The model under review builds one solid part; all positions refer to its coordinate system, in mm. A direction names the side the tool comes from. Coordinates: 2 decimals unless noted, no trailing zeros. Loops run counter-clockwise (first coordinate to the right, second up) from the corner with the lowest first, then second, coordinate; pieces in that order, holes last. Notation, with made-up numbers: M 58.25,49.25 L 80.25,49.25 A23 ccw 80.25,57.25 Z; hole C 27.25,16.25 d7. An arc over 180 degrees is marked long. Use CSV: the item, a comma, the result in double quotes. Start each with the question number.
1. Tool access review of faces 1 (the flat face through (7, 7, 0)), 2 (the flat face through (0.125, -11, 3)): name each direction out of +Z, -Z, +X, -X, +Y, -Y from which nothing blocks a thin tool from reaching the whole face with its end or side.
2. For L1, parallel to X at y = -5.25, z = 2.6; L2, parallel to Y at x = 3.5, z = 0.6; L3, parallel to X at y = 0, z = 1 (3 decimals), list the stretches that pass through material, from the lowest coordinate up.
3. Clearance check with flat-ended pins moving along their axes: P1, Ø9.5, axis at x = 2.5, y = -2, coming from the +Z side; P2, Ø1, axis at y = -7.5, z = 2, coming from the -X side; P3, Ø2.5, axis at y = -11, z = 1.5, coming from the +X side; P4, Ø2.5, axis at y = -11, z = 3, coming from the -X side. State where each tip first meets the part, or that it passes through.
4. Add section A-A, the plane z = 1.2. Write out the cut boundary in (x, y) (3 decimals), then the cut area to 3 significant figures.
from build123d import *

# Parameters (mm, degrees)
F0_R      = 12.5
F0_R_2    = 9.625
F1_DEPTH  = 4.95
F2_R      = 2.25
F4_R      = 9.625
F4_R_2    = 9.5
F5_DEPTH  = 0.2
F7_R      = 9.625
F7_R_2    = 9.5
F8_DEPTH  = 0.4
F11_DEPTH = 0.4
F12_DEPTH = 25


with BuildPart() as f1:
    # F0 (on Top) → F1 (new body)
    with BuildSketch(Plane.XY):
        Circle(F0_R)
        Circle(F0_R_2, mode=Mode.SUBTRACT)
    extrude(amount=F1_DEPTH)

    # F2
    f2_edges = [f1.edges().sort_by_distance(p)[0] for p in [
        (-12.5, 0, 4.95),
        (-12.5, 0, 0),
    ]]
    fillet(f2_edges, radius=F2_R)

    # F4 (on offset) → F5 (join, symmetric)
    with BuildSketch(Plane.XY.offset(2.475)):
        Circle(F4_R)
        Circle(F4_R_2, mode=Mode.SUBTRACT)
    extrude(amount=F5_DEPTH, both=True)

    # F7 (on offset) → F8 (join)
    with BuildSketch(Plane(origin=(0, 0, 0), x_dir=(1, 0, 0), z_dir=(0, 0, -1))):
        Circle(F7_R)
        Circle(F7_R_2, mode=Mode.SUBTRACT)
    extrude(amount=-F8_DEPTH)

    # F10 (on offset) → F11 (join)
    with BuildSketch(Plane.XY.offset(4.95)):
        with BuildLine():
            ThreePointArc((0.125, -9.499177596), (0, -9.5), (-0.125, -9.499177596))
            Line((-0.125, -9.499177596), (-0.125, -9.6241882775))
            ThreePointArc((-0.125, -9.6241882775), (0, -9.625), (0.125, -9.6241882775))
            Line((0.125, -9.6241882775), (0.125, -9.499177596))
        make_face()
        with BuildLine():
            ThreePointArc((-0.125, -9.499177596), (-6.6731739075, 6.7615641681), (9.5, 0))
            ThreePointArc((9.5, 0), (6.7615641681, -6.6731739075), (0.125, -9.499177596))
            Line((0.125, -9.499177596), (0.125, -9.6241882775))
            ThreePointArc((0.125, -9.6241882775), (6.8499543794, -6.7615641681), (9.625, 0))
            ThreePointArc((9.625, 0), (-6.7615641681, 6.8499543794), (-0.125, -9.6241882775))
            Line((-0.125, -9.6241882775), (-0.125, -9.499177596))
        make_face()
    extrude(amount=-F11_DEPTH)

    # F10 (on offset) → F12 (cut)
    with BuildSketch(Plane.XY.offset(4.95)):
        with BuildLine():
            ThreePointArc((0.125, -9.6241882775), (0, -9.625), (-0.125, -9.6241882775))
            Line((-0.125, -9.6241882775), (-0.125, -12.8121394664))
            Line((-0.125, -12.8121394664), (0.125, -12.8121394664))
            Line((0.125, -12.8121394664), (0.125, -9.6241882775))
        make_face()
        with BuildLine():
            ThreePointArc((0.125, -9.499177596), (0, -9.5), (-0.125, -9.499177596))
            Line((-0.125, -9.499177596), (-0.125, -9.6241882775))
            ThreePointArc((-0.125, -9.6241882775), (0, -9.625), (0.125, -9.6241882775))
            Line((0.125, -9.6241882775), (0.125, -9.499177596))
        make_face()
        with BuildLine():
            Line((-0.125, -8.5825398564), (-0.125, -9.499177596))
            ThreePointArc((-0.125, -9.499177596), (0, -9.5), (0.125, -9.499177596))
            Line((0.125, -9.499177596), (0.125, -8.5825398564))
            Line((0.125, -8.5825398564), (-0.125, -8.5825398564))
        make_face()
    extrude(amount=-F12_DEPTH, mode=Mode.SUBTRACT)


solid = f1.part
Computed:
1,face 1,"-Z, +X, -X, +Y, -Y"
1,face 2,"+Z, -Z, -Y"
2,L1,"x = -11.34 to -7.92, 7.92 to 11.34"
2,L2,"y = -11.25 to -8.97, 8.97 to 11.25"
2,L3,"x = -12.121 to -9.625, 9.625 to 12.121"
3,P1,"passes through"
3,P2,"stops at x = -10.34"
3,P3,"stops at x = 7.7"
3,P4,"stops at x = -7.8"
4,outline,"M -0.125,-12.239 L -0.125,-9.624 A9.625 cw long 0.125,-9.624 L 0.125,-12.239 A12.24 ccw long Z"
4,area,"179 mm^2"
